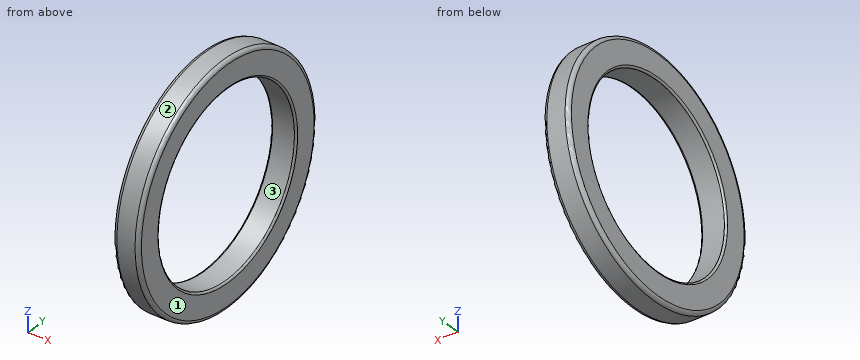
from build123d import *

# Parameters (mm, degrees)
SKETCH1_R           = 32.5
SKETCH1_R_2         = 25
BOSS_EXTRUDE1_DEPTH = 7
FILLET1_R           = 1
FILLET2_R           = 0.5


with BuildPart() as part:
    # Sketch1 → Boss-Extrude1 (new body)
    with BuildSketch(Plane(origin=(0, 0, 0), x_dir=(0, 0, -1), z_dir=(1, 0, 0))):
        Circle(SKETCH1_R)
        Circle(SKETCH1_R_2, mode=Mode.SUBTRACT)
    extrude(amount=BOSS_EXTRUDE1_DEPTH)

    # Fillet1
    fillet1_edges = [part.edges().sort_by_distance(p)[0] for p in [
        (0, 0, 32.5),
        (7, 0, 32.5),
    ]]
    fillet(fillet1_edges, radius=FILLET1_R)

    # Fillet2
    fillet2_edges = [part.edges().sort_by_distance(p)[0] for p in [
        (0, 0, 25),
        (7, 0, 25),
    ]]
    fillet(fillet2_edges, radius=FILLET2_R)


solid = part.part
Check sheet for the modelled part. Datum: model origin and axes. Units: mm. Face numbers are marked on the shaded views. Round coordinates to 2 decimals unless told otherwise and drop trailing zeros. Loops run counter-clockwise (first coordinate to the right, second up) from the corner with the lowest first, then second, coordinate; pieces in that order, holes last. Notation, with made-up numbers: (20, -32) -> (58, -32) arc R20 cw to (58, -8) -> close; hole circle Ø6 at (-39, 37). An arc over 180 degrees is marked (long way). Put each result on its own line as item: value. Start each with the question number.
1. Draft check along Z on the marked faces 1, 2 and 3. Enter one of: +Z half, -Z half, draft (parallel to the pull), parting line (faces both ways), or undercut.
2. Gauge pin test, flat ends, axial feed: pin 1 (12 mm diameter, centred on y = 15, z = -17, fed in from -X); pin 2 (3 mm diameter, centred on x = 3.5, z = -4, fed in from +Y). Record the tip position at first contact, or that the pin passes through.
3. Scan lines: probe 1 along Y at (x, z) = (1.7, 0); probe 2 along Y at (x, z) = (2, -10.5); probe 3 along Z at (x, y) = (4, 17). Record each from-to range of solid material in increasing order.
4. Section check C-C (x = 4.5). Enter the section's corners in (y, z), plus the area to 3 significant figures.
5. Section check A-A (y = 0). Enter the section's corners in (x, z), plus the area to 3 significant figures.
Findings:
1. face 1: draft
1. face 2: parting line
1. face 3: undercut
2. pin 1: stops at x = 0
2. pin 2: stops at y = 32.4
3. probe 1: y = -32.5 to -25, 25 to 32.5
3. probe 2: y = -30.76 to -22.69, 22.69 to 30.76
3. probe 3: z = -27.7 to -18.33, 18.33 to 27.7
4. outline: circle Ø65 at (0, 0); hole circle Ø50 at (0, 0)
4. area: 1,350 mm^2
5. outline: (0, -31.5) arc R1 ccw to (1, -32.5) -> (6, -32.5) arc R1 ccw to (7, -31.5) -> (7, -25.5) arc R0.5 ccw to (6.5, -25) -> (0.5, -25) arc R0.5 ccw to (0, -25.5) -> close; (0, 25.5) arc R0.5 ccw to (0.5, 25) -> (6.5, 25) arc R0.5 ccw to (7, 25.5) -> (7, 31.5) arc R1 ccw to (6, 32.5) -> (1, 32.5) arc R1 ccw to (0, 31.5) -> close
5. area: 104 mm^2
